Drawing for the job (mm, zero at the part's lowest x, y, z). A direction names the side the tool comes from. Coordinates: 2 decimals unless noted, no trailing zeros. Order: outer loops, then holes, each group sorted by start corner. A loop starts at its lowest first (then second) coordinate and runs counter-clockwise, first axis right, second up.
1) Cut at D-D (y = 1.5). List the corners of the cut face in (x, z).
2) Wall check: L1, parallel to Z at x = 7.5, y = 7.25; L2, parallel to Z at x = 1.5, y = 11.75; L3, parallel to X at y = 4.5, z = 32. Give the ranges that are in metal, low to high.
3) Tool access for the marked faces 1 and 2: list every direction of +Z, -Z, +X, -X, +Y, -Y with a clear straight run to the whole face (end or side of a thin tool).
4) Cut at C-C (x = 3). List the corners of the cut face in (y, z).
5) Cut at A-A (x = 7.5). List the corners of the cut face in (y, z).
6) Pin check, flat tips, straight feed: pin 1 Ø4 at (x, z) = (4.5, 10) entering from +Y; pin 2 Ø1.2 at (x, z) = (7.5, 32) entering from -Y; pin 3 Ø8 at (x, z) = (5, 22) entering from -Y; pin 4 Ø5 at (x, z) = (1.5, 11.5) entering from -Y. Stop position of each tip, or through.
7) Cut at B-B (y = 7.5). List the corners of the cut face in (x, z).
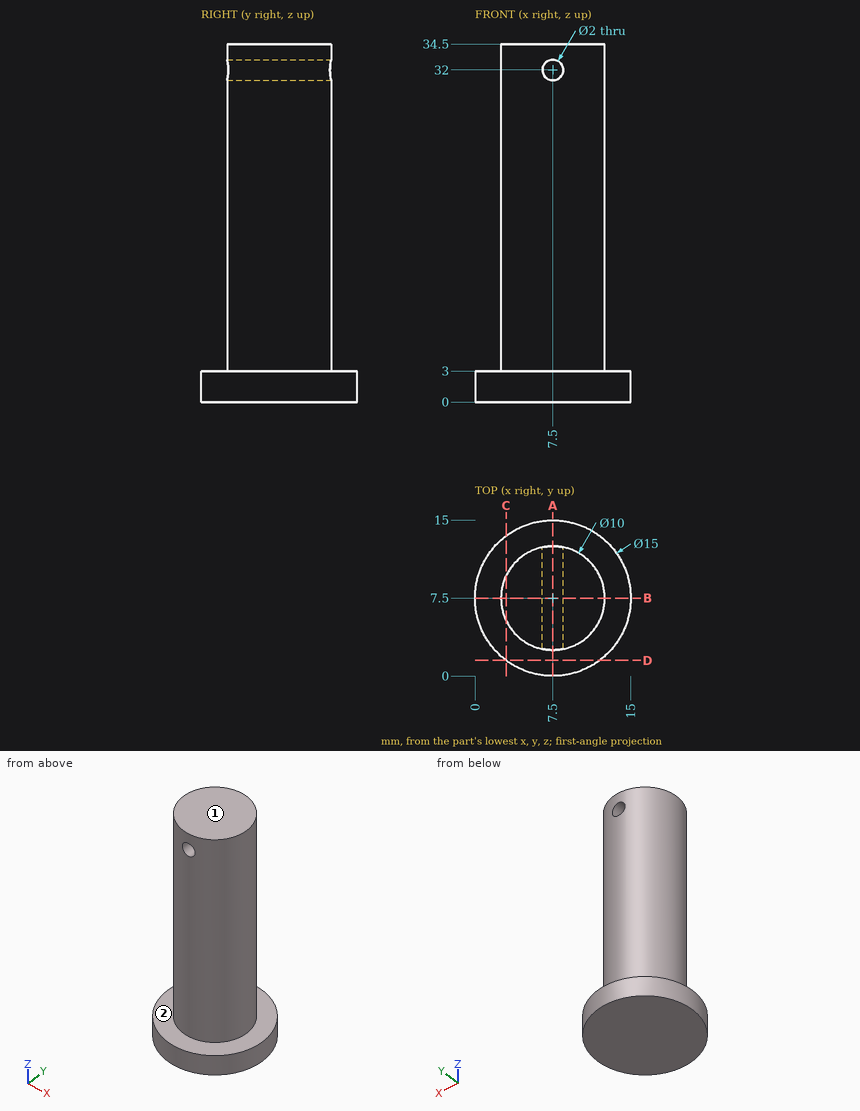
Geometry check:
1. outline: (3, 0) - (12, 0) - (12, 3) - (3, 3) - close
2. L1: z = 0 to 31, 33 to 34.5
2. L2: z = 0 to 3
2. L3: x = 3.5 to 6.5, 8.5 to 11.5
3. face 1: +Z, +X, -X, +Y, -Y
3. face 2: +Z
4. outline: (1.5, 0) - (13.5, 0) - (13.5, 3) - (9.68, 3) - (9.68, 34.5) - (5.32, 34.5) - (5.32, 3) - (1.5, 3) - close
5. outline: (0, 0) - (15, 0) - (15, 3) - (12.5, 3) - (12.5, 31) - (2.5, 31) - (2.5, 3) - (0, 3) - close; (2.5, 33) - (12.5, 33) - (12.5, 34.5) - (2.5, 34.5) - close
6. pin 1: stops at y = 12.4
6. pin 2: passes through
6. pin 3: stops at y = 2.5
6. pin 4: stops at y = 3.93
7. outline: (0, 0) - (15, 0) - (15, 3) - (12.5, 3) - (12.5, 34.5) - (2.5, 34.5) - (2.5, 3) - (0, 3) - close; hole circle Ø2 at (7.5, 32)
